```python
from build123d import *

# Parameters (mm, degrees)
F0_W     = 140
F0_H     = 220
F0_R     = 2.25
F1_DEPTH = 2
F2_W     = 2
F2_H     = 2
F2_R     = 1.75
F3_DEPTH = 2
F4_R     = 3
F5_R     = 1.5


with BuildPart() as f1:
    # F0 (on Front) → F1 (new body)
    with BuildSketch(Plane.XZ):
        with Locations((70, 110)):
            Rectangle(F0_W, F0_H)
        with Locations((5, 5)):
            Circle(F0_R, mode=Mode.SUBTRACT)
        with Locations((135, 5)):
            Circle(F0_R, mode=Mode.SUBTRACT)
        with Locations((5, 112.5)):
            Circle(F0_R, mode=Mode.SUBTRACT)
        with Locations((5, 215)):
            Circle(F0_R, mode=Mode.SUBTRACT)
        with Locations((135, 112.5)):
            Circle(F0_R, mode=Mode.SUBTRACT)
        with Locations((135, 215)):
            Circle(F0_R, mode=Mode.SUBTRACT)
    extrude(amount=F1_DEPTH)

    # F2 (on face) → F3 (cut)
    with BuildSketch(Plane.XZ.offset(2)):
        with Locations((21, 111)):
            Rectangle(F2_W, F2_H)
        with Locations((19, 111)):
            Rectangle(F2_W, F2_H)
        with BuildLine():
            Line((18, 112), (20, 112))
            Line((20, 112), (22, 112))
            Line((22, 112), (22, 117.5))
            ThreePointArc((22, 117.5), (20, 119.5), (18, 117.5))
            Line((18, 117.5), (18, 112))
        make_face()
        with Locations((21, 109)):
            Rectangle(F2_W, F2_H)
        with Locations((19, 109)):
            Rectangle(F2_W, F2_H)
        with BuildLine():
            Line((18, 110), (18, 112))
            Line((18, 112), (12.5, 112))
            ThreePointArc((12.5, 112), (10.5, 110), (12.5, 108))
            Line((12.5, 108), (18, 108))
            Line((18, 108), (18, 110))
        make_face()
        with BuildLine():
            Line((27.5, 112), (22, 112))
            Line((22, 112), (22, 110))
            Line((22, 110), (22, 108))
            Line((22, 108), (27.5, 108))
            ThreePointArc((27.5, 108), (29.5, 110), (27.5, 112))
        make_face()
        with BuildLine():
            Line((22, 108), (20, 108))
            Line((20, 108), (18, 108))
            Line((18, 108), (18, 102.5))
            ThreePointArc((18, 102.5), (20, 100.5), (22, 102.5))
            Line((22, 102.5), (22, 108))
        make_face()
        with Locations((121, 111)):
            Rectangle(F2_W, F2_H)
        with Locations((119, 111)):
            Rectangle(F2_W, F2_H)
        with BuildLine():
            Line((118, 112), (120, 112))
            Line((120, 112), (122, 112))
            Line((122, 112), (122, 117.5))
            ThreePointArc((122, 117.5), (120, 119.5), (118, 117.5))
            Line((118, 117.5), (118, 112))
        make_face()
        with Locations((121, 109)):
            Rectangle(F2_W, F2_H)
        with Locations((119, 109)):
            Rectangle(F2_W, F2_H)
        with BuildLine():
            Line((118, 110), (118, 112))
            Line((118, 112), (112.5, 112))
            ThreePointArc((112.5, 112), (110.5, 110), (112.5, 108))
            Line((112.5, 108), (118, 108))
            Line((118, 108), (118, 110))
        make_face()
        with BuildLine():
            Line((127.5, 112), (122, 112))
            Line((122, 112), (122, 110))
            Line((122, 110), (122, 108))
            Line((122, 108), (127.5, 108))
            ThreePointArc((127.5, 108), (129.5, 110), (127.5, 112))
        make_face()
        with BuildLine():
            Line((122, 108), (120, 108))
            Line((120, 108), (118, 108))
            Line((118, 108), (118, 102.5))
            ThreePointArc((118, 102.5), (120, 100.5), (122, 102.5))
            Line((122, 102.5), (122, 108))
        make_face()
        with Locations((70, 110)):
            Circle(F2_R)
        with Locations((71, 161)):
            Rectangle(F2_W, F2_H)
        with BuildLine():
            Line((68, 162), (70, 162))
            Line((70, 162), (72, 162))
            Line((72, 162), (72, 167.5))
            ThreePointArc((72, 167.5), (70, 169.5), (68, 167.5))
            Line((68, 167.5), (68, 162))
        make_face()
        with Locations((69, 161)):
            Rectangle(F2_W, F2_H)
        with Locations((71, 159)):
            Rectangle(F2_W, F2_H)
        with Locations((69, 159)):
            Rectangle(F2_W, F2_H)
        with BuildLine():
            Line((77.5, 162), (72, 162))
            Line((72, 162), (72, 160))
            Line((72, 160), (72, 158))
            Line((72, 158), (77.5, 158))
            ThreePointArc((77.5, 158), (79.5, 160), (77.5, 162))
        make_face()
        with BuildLine():
            Line((68, 160), (68, 162))
            Line((68, 162), (62.5, 162))
            ThreePointArc((62.5, 162), (60.5, 160), (62.5, 158))
            Line((62.5, 158), (68, 158))
            Line((68, 158), (68, 160))
        make_face()
        with BuildLine():
            Line((72, 158), (70, 158))
            Line((70, 158), (68, 158))
            Line((68, 158), (68, 152.5))
            ThreePointArc((68, 152.5), (70, 150.5), (72, 152.5))
            Line((72, 152.5), (72, 158))
        make_face()
        with BuildLine():
            ThreePointArc((77.5, 58), (79.5, 60), (77.5, 62))
            Line((77.5, 62), (72, 62))
            Line((72, 62), (72, 60))
            Line((72, 60), (72, 58))
            Line((72, 58), (77.5, 58))
        make_face()
        with Locations((71, 61)):
            Rectangle(F2_W, F2_H)
        with BuildLine():
            Line((70, 62), (72, 62))
            Line((72, 62), (72, 67.5))
            ThreePointArc((72, 67.5), (70, 69.5), (68, 67.5))
            Line((68, 67.5), (68, 62))
            Line((68, 62), (70, 62))
        make_face()
        with Locations((69, 61)):
            Rectangle(F2_W, F2_H)
        with Locations((71, 59)):
            Rectangle(F2_W, F2_H)
        with BuildLine():
            Line((72, 52.5), (72, 58))
            Line((72, 58), (70, 58))
            Line((70, 58), (68, 58))
            Line((68, 58), (68, 52.5))
            ThreePointArc((68, 52.5), (70, 50.5), (72, 52.5))
        make_face()
        with BuildLine():
            Line((68, 60), (68, 62))
            Line((68, 62), (62.5, 62))
            ThreePointArc((62.5, 62), (60.5, 60), (62.5, 58))
            Line((62.5, 58), (68, 58))
            Line((68, 58), (68, 60))
        make_face()
        with Locations((69, 59)):
            Rectangle(F2_W, F2_H)
    extrude(amount=-F3_DEPTH, mode=Mode.SUBTRACT)

    # F4
    f4_edges = [f1.edges().sort_by_distance(p)[0] for p in [
        (18, -1, 112),
        (22, -1, 112),
        (18, -1, 108),
        (22, -1, 108),
        (118, -1, 112),
        (122, -1, 112),
        (118, -1, 108),
        (122, -1, 108),
    ]]
    fillet(f4_edges, radius=F4_R)

    # F5
    f5_edges = [f1.edges().sort_by_distance(p)[0] for p in [
        (0, -1, 220),
        (140, -1, 220),
        (0, -1, 0),
        (140, -1, 0),
    ]]
    fillet(f5_edges, radius=F5_R)


solid = f1.part
```
Verification items for the finished model (mm, model axes). Round coordinates to 2 decimals unless told otherwise and drop trailing zeros. Put each result on its own line as item: value. Start each with the question number.
(1) Draft check along Z on faces 1 (the face through (69, 0, 112)), 2 (the face through (137.146, -0.986, 5.676)). Enter one of: +Z half, -Z half, draft (parallel to the pull), parting line (faces both ways), or undercut.
(2) Section check A-A (y = -1.4). State how many separate pieces and enclosed holes the cut face has, then the cut area to 3 significant figures.
(3) Material ranges on line 1 along X through (y, z) = (-0.45, 110); line 2 along Z through (x, y) = (135, -0.9); line 3 along Z through (x, y) = (70, -1.3), recorded low to high.
(4) Depth check by flat-ended pin: pin 1 Ø3.5 at (x, z) = (135, 112.5) entering from +Y. Enter the tip coordinate at first touch or a pass-through.
Completed:
1. face 1: draft
1. face 2: undercut
2. separate pieces: 1
2. enclosed holes: 11
2. area: 30,200 mm2
3. line 1: x = 0 to 10.5, 29.5 to 68.25, 71.75 to 110.5, 129.5 to 140
3. line 2: z = 0 to 2.75, 7.25 to 110.25, 114.75 to 212.75, 217.25 to 220
3. line 3: z = 0 to 50.5, 69.5 to 108.25, 111.75 to 150.5, 169.5 to 220
4. pin 1: passes through
